from build123d import *

# Parameters (mm, degrees)
F0_R      = 8
F1_DEPTH  = 60
F3_DEPTH  = 50.001
F4_W      = 20
F4_H      = 50
F5_DEPTH  = 60
F7_DEPTH  = 60.001
F9_DEPTH  = 50.001
F13_DEPTH = 50.001
F11_W     = 20.90599
F11_H     = 10.90599
F12_DEPTH = 100.001


with BuildPart() as f1:
    # F0 (on Front) → F1 (new body)
    with BuildSketch(Plane.XZ):
        with BuildLine():
            Line((-80, 0), (0, 0))
            Line((0, 0), (0, 50))
            Line((0, 50), (-21.90525, 50))
            ThreePointArc((-21.90525, 50), (-53.528026, 43.484692), (-80, 25))
            Line((-80, 25), (-80, 0))
        make_face()
        with Locations((-40, 25)):
            Circle(F0_R, mode=Mode.SUBTRACT)
    extrude(amount=-F1_DEPTH)

    # F2 (on Top) → F3 (cut, through all)
    with BuildSketch(Plane.XY):
        Polygon((-15, 30), (-80, 30), (-80, 10), (-65, 10), (-65, 15), (-15, 15), align=None)
        Polygon((-80, 50), (-80, 30), (-15, 30), (-15, 45), (-65, 45), (-65, 50), align=None)
    extrude(amount=F3_DEPTH, mode=Mode.SUBTRACT)

    # F4 (on Front) → F5 (join)
    with BuildSketch(Plane.XZ):
        with Locations((10, 25)):
            Rectangle(F4_W, F4_H)
    extrude(amount=-F5_DEPTH)

    # F6 (on Front) → F7 (cut, through all)
    with BuildSketch(Plane.XZ):
        Polygon((20, 50), (0, 50), (20, 38.452995), align=None)
        Polygon((20, 11.547005), (0, 0), (20, 0), align=None)
    extrude(amount=-F7_DEPTH, mode=Mode.SUBTRACT)

    # F8 (on face) → F9 (cut, through all)
    with BuildSketch(Plane.XY.offset(50)):
        Polygon((20, 11.547005), (0, 0), (20, 0), align=None)
        Polygon((20, 60), (0, 60), (20, 48.452995), align=None)
    extrude(amount=-F9_DEPTH, mode=Mode.SUBTRACT)

    # F10 (on Top) → F13 (cut, through all)
    with BuildSketch(Plane.XY):
        Polygon((20, 11.547005), (0, 0), (20, 0), align=None)
        Polygon((20, 60), (0, 60), (20, 48.452995), align=None)
    extrude(amount=F13_DEPTH, mode=Mode.SUBTRACT)

    # F11 (on face) → F12 (cut, through all)
    with BuildSketch(Plane.YZ.offset(20)):
        with Locations((30, 25)):
            Rectangle(F11_W, F11_H)
    extrude(amount=-F12_DEPTH, mode=Mode.SUBTRACT)


solid = f1.part
Verification items for the finished model (mm, model axes). A direction names the side the tool comes from. Coordinates: 2 decimals unless noted, no trailing zeros. Write each loop counter-clockwise with the first axis right and the second up, starting at its lowest first coordinate (ties: lowest second). Pieces come first, ordered by that corner, then holes. Notation, with made-up numbers: (81, 16.25) -> (119, 16.25) arc R14 cw to (119, 40.25) -> close; hole circle Ø6 at (61.5, -16). An arc over 180 degrees is marked (long way). One line per item, written item: value. Start each with the question number.
Q1. Go/stop test with flat-tipped pins: P1, Ø5, axis at y = 21.5, z = 7, coming from the -X side; P2, Ø3.5, axis at x = 10.5, z = 26, coming from the -Y side; P3, Ø5, axis at y = 9.5, z = 29, coming from the +X side; P4, Ø4, axis at y = 47, z = 11.5, coming from the -X side. Record where each tip stops, or that it passes through.
Q2. Access from +Z, -Z, +X, -X, +Y, -Y to the whole of each face (thin tool, end or side, straight path). Record for faces 1 (the flat face through (-46, 15, 19)), 2 (the flat face through (3, 30, 30.453)), 3 (the flat face through (-31.7, 0, 25.4)).
Q3. Thickness scan on L1, parallel to Y at x = -49.5, z = 41; L2, parallel to Z at x = -6.5, y = 28.5; L3, parallel to X at y = 28, z = 38. Record the ranges inside material, lowest first. Write a range as from..to.
Q4. Cross-section at C-C on x = -40. Enter the section's corners in (y, z).
Q5. Cross-section at A-A on x = -55. Enter the section's corners in (y, z).
Q6. Cross-section at B-B on z = 21. Enter the section's corners in (x, y).
Q7. Cross-section at D-D on x = -6.5. Enter the section's corners in (y, z).
Checked values:
1. P1: stops at x = -15
1. P2: stops at y = 5.05
1. P3: stops at x = 20
1. P4: stops at x = -65
2. face 1: +Z, -Z, -X
2. face 2: +X, -X
2. face 3: +Z, -Z, +X, -X, -Y
3. L1: y = 0..15, 45..60
3. L2: z = 0..19.55, 30.45..50
3. L3: x = -15..20
4. outline: (0, 0) -> (15, 0) -> (15, 17) -> (0, 17) -> close; (0, 33) -> (15, 33) -> (15, 47.93) -> (0, 47.93) -> close; (45, 0) -> (60, 0) -> (60, 17) -> (45, 17) -> close; (45, 33) -> (60, 33) -> (60, 47.93) -> (45, 47.93) -> close
5. outline: (0, 0) -> (15, 0) -> (15, 42.83) -> (0, 42.83) -> close; (45, 0) -> (60, 0) -> (60, 42.83) -> (45, 42.83) -> close
6. outline: (-80, 0) -> (-46.93, 0) -> (-46.93, 15) -> (-65, 15) -> (-65, 10) -> (-80, 10) -> close; (-80, 50) -> (-65, 50) -> (-65, 45) -> (-46.93, 45) -> (-46.93, 60) -> (-80, 60) -> close; (-33.07, 0) -> (0, 0) -> (20, 11.55) -> (20, 19.55) -> (-15, 19.55) -> (-15, 15) -> (-33.07, 15) -> close; (-33.07, 45) -> (-15, 45) -> (-15, 40.45) -> (20, 40.45) -> (20, 48.45) -> (0, 60) -> (-33.07, 60) -> close
7. outline: (0, 0) -> (60, 0) -> (60, 50) -> (0, 50) -> close; hole (19.55, 19.55) -> (40.45, 19.55) -> (40.45, 30.45) -> (19.55, 30.45) -> close
